Design review of the part built by this model. Coordinates are the model's own, in mm. Face numbers are marked on the shaded views. A direction names the side the tool comes from. Round coordinates to 2 decimals unless told otherwise and drop trailing zeros. Write each loop counter-clockwise with the first axis right and the second up, starting at its lowest first coordinate (ties: lowest second). Pieces come first, ordered by that corner, then holes. Notation, with made-up numbers: (67.25, -21) - (126.25, -21) arc R14 ccw to (126.25, 6) - close; hole circle Ø10 at (-23, 7.25). An arc over 180 degrees is marked (long way). Use one line per item in the form item = value.
```python
from build123d import *

# Parameters (mm, degrees)
SKETCH_W        = 50
SKETCH_H        = 44
PAD_DEPTH       = 5
SKETCH001_W     = 2.2
SKETCH001_H     = 2.3
POCKET_DEPTH    = 50.001
POCKET002_DEPTH = 50.001
SKETCH002_W     = 10
SKETCH002_H     = 28
POCKET001_DEPTH = 10.001
FILLET_R        = 1
FILLET001_R     = 0.5
CHAMFER_1_ANGLE = 30
CHAMFER_1_SIZE  = 1.3
CHAMFER_2_ANGLE = 30
CHAMFER_2_SIZE  = 1.3


with BuildPart() as part:
    # Sketch (on XY_Plane of Origin) → Pad (new body, symmetric)
    with BuildSketch(Plane.XY):
        Rectangle(SKETCH_W, SKETCH_H)
    extrude(amount=PAD_DEPTH, both=True)

    # Sketch001 (on Face2 of Pad) → Pocket (cut, through all)
    with BuildSketch(Plane.YZ.offset(25)):
        Polygon((0.25, 5), (0.25, 3.5), (-0.25, 2.5), (-0.25, 0), (16, 0), (16, 2.5), (15.5, 3.5), (15.5, 5), align=None)
        with Locations((-17, 1.5)):
            Rectangle(SKETCH001_W, SKETCH001_H)
    extrude(amount=-POCKET_DEPTH, mode=Mode.SUBTRACT)

    # Sketch003 (on Face3 of Pocket) → Pocket002 (cut, through all)
    with BuildSketch(Plane.YZ.offset(25)):
        with BuildLine():
            ThreePointArc((16, 0), (15, 1), (14, 0))
            Line((14, 0), (14, -2.5))
            ThreePointArc((14, -2.5), (15, -3.5), (16, -2.5))
            Line((16, 0), (16, -2.5))
        make_face()
    extrude(amount=-POCKET002_DEPTH, mode=Mode.SUBTRACT)

    # Sketch002 (on Face4 of Pocket) → Pocket001 (cut, through all)
    with BuildSketch(Plane(origin=(0, 0, -5), x_dir=(1, 0, 0), z_dir=(0, 0, -1))):
        with Locations((20, -8)):
            Rectangle(SKETCH002_W, SKETCH002_H)
    extrude(amount=-POCKET001_DEPTH, mode=Mode.SUBTRACT)

    # Fillet
    fillet_edges = [part.edges().sort_by_distance(p)[0] for p in [
        (25, -22, 0),
        (25, -6, 0),
        (-25, -22, 0),
        (15, 22, 0),
        (15, -6, 0),
        (-25, 22, 0),
    ]]
    fillet(fillet_edges, radius=FILLET_R)

    # Fillet001
    fillet001_edges = [part.edges().sort_by_distance(p)[0] for p in [
        (-25, -15.9, 1.5),
        (-25, -18.1, 1.5),
        (25, -15.9, 1.5),
        (25, -18.1, 1.5),
        (15, 14, -1.25),
        (-25, 14, -1.25),
    ]]
    fillet(fillet001_edges, radius=FILLET001_R)

    # Chamfer 1
    chamfer_1_edges = [part.edges().sort_by_distance(p)[0] for p in [
        (-5, 15.5, 5),
    ]]
    chamfer_1_side = part.faces().sort_by_distance((-5, 15.5, 4.25))[0]
    chamfer(chamfer_1_edges, length=CHAMFER_1_SIZE, angle=CHAMFER_1_ANGLE, reference=chamfer_1_side)

    # Chamfer 2
    chamfer_2_edges = [part.edges().sort_by_distance(p)[0] for p in [
        (-5, 0.25, 5),
    ]]
    chamfer_2_side = part.faces().sort_by_distance((-5, 0.25, 4.25))[0]
    chamfer(chamfer_2_edges, length=CHAMFER_2_SIZE, angle=CHAMFER_2_ANGLE, reference=chamfer_2_side)


solid = part.part
```
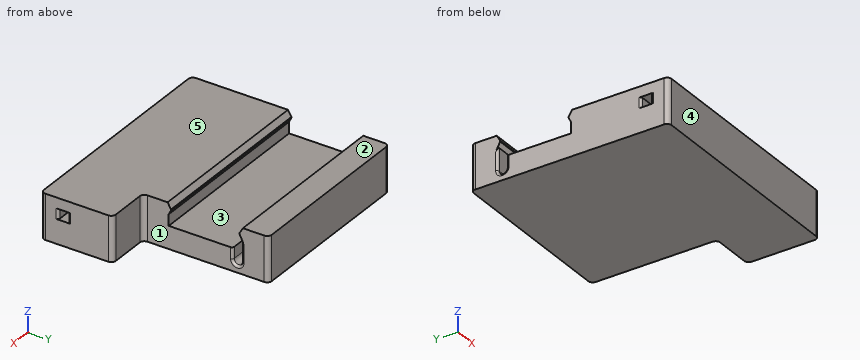
Q1. For P1, Ø11.5, axis at x = 0.5, y = 3.5, coming from the +Z side, flat-tipped, find the tip position at first contact; note if it passes through.
Calculated:
P1 = 5
Q2. We need section B-B on x = -4.5. Write out the cut boundary in (y, z).
Calculated:
outline = (-22, -5) - (22, -5) - (22, 5) - (16.25, 5) - (15.5, 3.7) - (15.5, 3.5) - (16, 2.5) - (16, -2.5) arc R1 cw to (14, -2.5) - (14, 0) - (-0.25, 0) - (-0.25, 2.5) - (0.25, 3.5) - (0.25, 3.7) - (-0.5, 5) - (-22, 5) - close; hole (-18.1, 0.35) - (-15.9, 0.35) - (-15.9, 2.65) - (-18.1, 2.65) - close
Q3. Machinability: for the marked faces 1 and 2, which of the approach directions +Z, -Z, +X, -X, +Y, -Y give a long, thin tool a straight path to every point of the face, cutting with its end or side? Answer none if there is none.
Calculated:
face_1 = +Z, -Z, +X, +Y
face_2 = +Z, +X, -X, +Y, -Y
Q4. To check wall thickness, follow line 1 along Y through (x, z) = (8.5, 1.5); line 2 along Y through (x, z) = (7, -0.25); line 3 along X through (y, z) = (-3.5, -0.5). State the ranges of each line that lie inside material, in increasing order. Write a range as from..to.
Calculated:
line_1 = -22..-18.1, -15.9..-0.25, 16..22
line_2 = -22..14, 16..22
line_3 = -25..15
Q5. Draft analysis for pull direction Y (two halves, no side actions). For the marked faces 3, 4 and 5, state which applies: released by +Y, released by -Y, zero draft, split by the parting line, or undercut.
Calculated:
face_3 = undercut
face_4 = released by -Y
face_5 = zero draft
Q6. We need section A-A on z = -1.75. Write out the cut boundary in (x, y), then the cut area to 3 significant figures.
Calculated:
outline = (-25, -21) arc R1 ccw to (-24, -22) - (24, -22) arc R1 ccw to (25, -21) - (25, -7) arc R1 ccw to (24, -6) - (16, -6) arc R1 cw to (15, -5) - (15, 13.5) arc R0.5 ccw to (14.5, 14) - (-24.5, 14) arc R0.5 ccw to (-25, 13.5) - close; (-25, 16.5) arc R0.5 ccw to (-24.5, 16) - (14.5, 16) arc R0.5 ccw to (15, 16.5) - (15, 21) arc R1 ccw to (14, 22) - (-24, 22) arc R1 ccw to (-25, 21) - close
area = 1,840 mm2
Q7. We need section D-D on y = 5. Write out the cut boundary in (x, z).
Calculated:
outline = (-25, -5) - (15, -5) - (15, 0) - (-25, 0) - close
Q8. We need section C-C on x = 17. Write out the cut boundary in (y, z).
Calculated:
outline = (-22, -5) - (-6, -5) - (-6, 5) - (-22, 5) - close; hole (-18.1, 0.35) - (-15.9, 0.35) - (-15.9, 2.65) - (-18.1, 2.65) - close
